Part print with two shaded views. Sizes in mm from the minimum x, y, z corner. A direction names the side the tool comes from. Coordinates: 2 decimals unless noted, no trailing zeros. Write each loop counter-clockwise with the first axis right and the second up, starting at its lowest first coordinate (ties: lowest second). Pieces come first, ordered by that corner, then holes. Notation, with made-up numbers: M -30.5,42 L 25.5,42 A18 cw 25.5,75 Z; hole C 68.5,51.25 d11. An arc over 180 degrees is marked long. Answer in a Markdown table with one row per item. Add a question column.
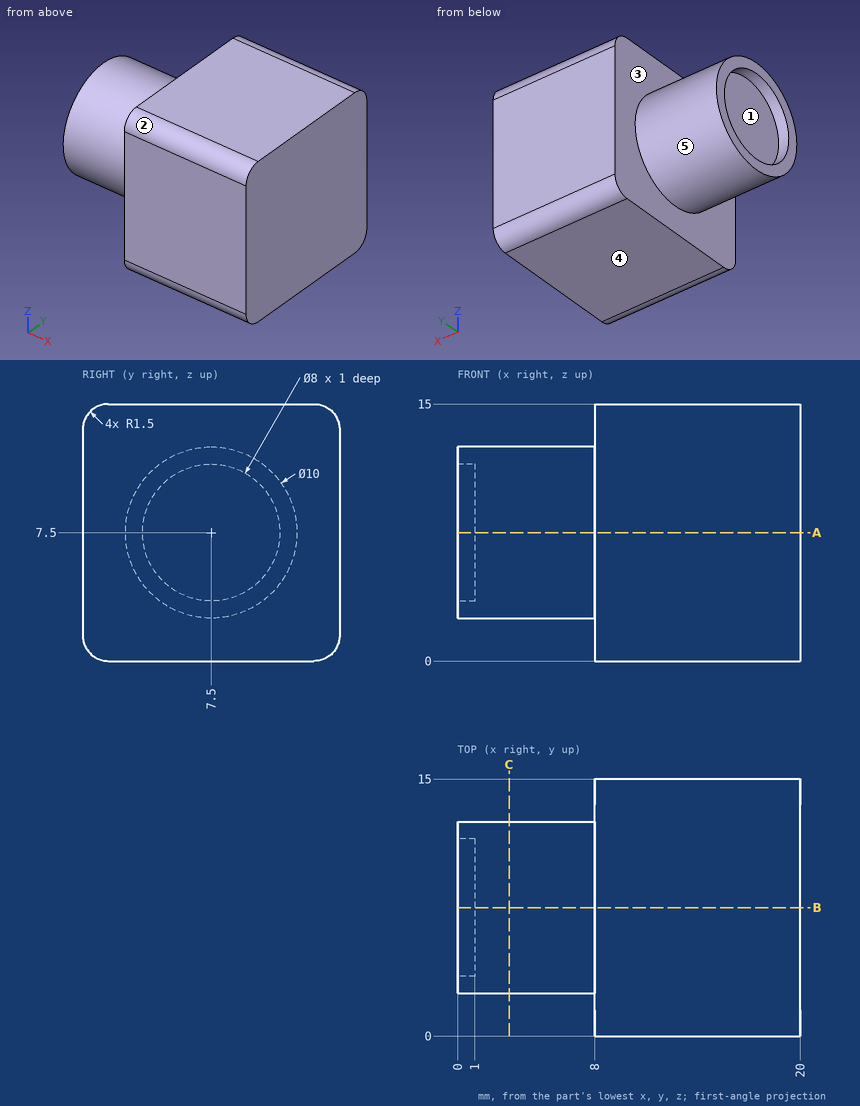
1) Slice it at C-C (x = 3). Give the cut face in (y, z), then the cut area to 3 significant figures.
2) Slice it at A-A (z = 7.5). Give the cut face in (x, y), then the cut area to 3 significant figures.
3) Two-plate mould, pull along Z, no slides. Class the marked faces 1, 2 and 3: released by +Z, released by -Z, zero draft, split by the parting line, or undercut.
4) Drill centre lines: probe 1 along Y at (x, z) = (0.35, 7.5); probe 2 along X at (y, z) = (14.25, 12.25); probe 3 along X at (y, z) = (10.5, 10). Where is each one in solid material? Low to high.
5) Which spindle directions (+Z, -Z, +X, -X, +Y, -Y) get a long thin tool onto all of the face, cutting with end or side? Do the marked faces 4 and 5. Say none if no direction does.
Ans:
| question | item | result |
|---|---|---|
| 1 | outline | C 7.5,7.5 d10 |
| 1 | area | 78.5 mm2 |
| 2 | outline | M 0,2.5 L 8,2.5 L 8,0 L 20,0 L 20,15 L 8,15 L 8,12.5 L 0,12.5 L 0,11.5 L 1,11.5 L 1,3.5 L 0,3.5 Z |
| 2 | area | 252 mm2 |
| 3 | face 1 | undercut |
| 3 | face 2 | released by +Z |
| 3 | face 3 | zero draft |
| 4 | probe 1 | y = 2.5 to 3.5, 11.5 to 12.5 |
| 4 | probe 2 | x = 8 to 20 |
| 4 | probe 3 | x = 1 to 20 |
| 5 | face 4 | -Z, +X, -X, +Y, -Y |
| 5 | face 5 | -X |
